Verification items for the finished model (mm, model axes). A direction names the side the tool comes from. Give positions to 0.01 mm unless a question says otherwise; leave off trailing zeros. Order: outer loops, then holes, each group sorted by start corner. A loop starts at its lowest first (then second) coordinate and runs counter-clockwise, first axis right, second up. Notation, with made-up numbers: M 69.25,-30.75 L 113.25,-30.75 A24 ccw 113.25,0.25 Z; hole C 81.25,-36 d7. An arc over 180 degrees is marked long. Answer as a JSON object with one key per item and string values.
```python
from build123d import *

# Parameters (mm, degrees)
BOSS_EXTRUDE1_DEPTH     = 13.28
CUT_EXTRUDE1_DEPTH      = 14.53406443
CUT_EXTRUDE1_DEPTH_BACK = 14.53406443
CUT_EXTRUDE5_DEPTH      = 0.29
CUT_EXTRUDE6_DEPTH      = 1.13
CUT_EXTRUDE7_DEPTH      = 0.87
CUT_EXTRUDE8_DEPTH      = 0.6


with BuildPart() as part:
    # Sketch1 → Boss-Extrude1 (new body)
    with BuildSketch(Plane.XY):
        Polygon((0, 0), (0, 2.28), (0.7, 2.28), (0.7, -0.58), (0, -0.58), (0, -1.88), (0.9, -1.88), (0.9, -2.45), (-0.7, -2.45), (-0.7, 0), align=None)
    extrude(amount=BOSS_EXTRUDE1_DEPTH)

    # Sketch2 → Cut-Extrude1 (cut, two sides)
    with BuildSketch(Plane(origin=(0, 0, 0), x_dir=(0, 0, -1), z_dir=(1, 0, 0))) as cut_extrude1_sk:
        Polygon((0.8, -2.75), (0.8, -0.085), (0.8, 2.58), (-2.665, 2.58), (0, -0.085), (-1.866053089, -2.75), align=None)
    extrude(amount=CUT_EXTRUDE1_DEPTH, mode=Mode.SUBTRACT)
    extrude(cut_extrude1_sk.sketch, amount=-CUT_EXTRUDE1_DEPTH_BACK, mode=Mode.SUBTRACT)

    # 3DSketch1 → Cut-Extrude5 (cut)
    with BuildSketch(Plane(origin=(0.7, 2.28, 7.8225), x_dir=(-0.5199469468957453, 0, -0.8541985556144386), z_dir=(0, 1, 0))):
        Polygon((0, 0), (0.982328339, -0.597938989), (1.346291202, 0), (0.363962863, 0.597938989), align=None)
    extrude(amount=-CUT_EXTRUDE5_DEPTH, mode=Mode.SUBTRACT)

    # 3DSketch1<3> → Cut-Extrude6 (cut)
    with BuildSketch(Plane(origin=(0, 2.28, 10.196397445), x_dir=(0.5199469468957453, 0, -0.8541985556144386), z_dir=(0, 1, 0))):
        Polygon((0, 0), (0.982328339, 0.597938989), (1.346291202, 0), (0.363962863, -0.597938989), align=None)
    extrude(amount=-CUT_EXTRUDE6_DEPTH, mode=Mode.SUBTRACT)

    # 3DSketch1<4> → Cut-Extrude7 (cut)
    with BuildSketch(Plane(origin=(0, 2.28, 5.478611146), x_dir=(0.519345577670118, 0, -0.8545643164528294), z_dir=(0, 1, 0))):
        Polygon((0, 0), (0.984308217, 0.598195022), (1.347850122, 0), (0.363541904, -0.598195022), align=None)
    extrude(amount=-CUT_EXTRUDE7_DEPTH, mode=Mode.SUBTRACT)

    # 3DSketch1<5> → Cut-Extrude8 (cut)
    with BuildSketch(Plane(origin=(0, 2.28, 3.471184381), x_dir=(0.5347339426738265, 0, -0.8450204793686985), z_dir=(0, 1, 0))):
        Polygon((0, 0), (0.934748456, 0.591514336), (1.309062216, 0), (0.37431376, -0.591514336), align=None)
    extrude(amount=-CUT_EXTRUDE8_DEPTH, mode=Mode.SUBTRACT)


solid = part.part
```
Q1. Tool access check on faces 4 (the face through (0.4, -1.88, 7.2)), 5 (the face through (0, 1, 7)), 6 (the face through (0.7, 1, 7)), 7 (the face through (0.3, -0.1, 13.28)), 8 (the face through (0, -2.45, 7)). Record the directions out of +Z, -Z, +X, -X, +Y, -Y that give a thin tool (end or side, any length) a straight path to the whole face; none if there is none.
Resolved:
{"face 4": "+Z, -Z, +X", "face 5": "+Z, -Z, -X, +Y", "face 6": "+Z, -Z, +X, +Y", "face 7": "+Z, +X, -X, +Y, -Y", "face 8": "+Z, -Z, +X, -X, -Y"}
Q2. Material ranges on L1, parallel to Z at x = 0.6, y = 1.6 (3 decimals); L2, parallel to Y at x = 0.25, z = 3.75; L3, parallel to Y at x = 0.1, z = 9.5, recorded low to high.
Resolved:
{"L1": "z = 1.685 to 4.327, 5.479 to 9.046, 10.196 to 13.28", "L2": "y = -2.45 to -1.88, -0.58 to 2.28", "L3": "y = -2.45 to -1.88, -0.58 to 1.15"}
Q3. Release check for a two-part mould opening along Y. For faces 1 (the face through (-0.267, -1.251, 0.816)), 2 (the face through (0, -1, 7)), 3 (the face through (-0.7, -1, 7)) record: +Y half, -Y half, draft (parallel to the pull), parting line (faces both ways), or undercut.
Resolved:
{"face 1": "-Y half", "face 2": "undercut", "face 3": "draft"}
Q4. Section check B-B on z = 4.75. Record the cut outline in (x, y).
Resolved:
{"outline": "M -0.7,-2.45 L 0.9,-2.45 L 0.9,-1.88 L 0,-1.88 L 0,-0.58 L 0.7,-0.58 L 0.7,1.41 L 0,1.41 L 0,0 L -0.7,0 Z"}
Q5. Gauge pin test, flat ends, axial feed: pin 1 Ø0.7 at (y, z) = (-1, 8) entering from +X; pin 2 Ø0.8 at (x, y) = (0, 2) entering from -Z (3 decimals); pin 3 Ø2 at (y, z) = (1, 5) entering from +X. Record the tip position at first contact, or that the pin passes through.
Resolved:
{"pin 1": "stops at x = 0", "pin 2": "stops at z = 1.685", "pin 3": "stops at x = 0.7"}
Q6. Section check C-C on z = 7.5. Record the cut outline in (x, y), then the cut area to 3 significant figures.
Resolved:
{"outline": "M -0.7,-2.45 L 0.9,-2.45 L 0.9,-1.88 L 0,-1.88 L 0,-0.58 L 0.7,-0.58 L 0.7,1.99 L 0,1.99 L 0,0 L -0.7,0 Z", "area": "4.03 mm²"}
Q7. Section check D-D on y = -0.75. Record the cut outline in (x, z).
Resolved:
{"outline": "M -0.7,0.47 L 0,0.47 L 0,13.28 L -0.7,13.28 Z"}
